For this review, take the finished solid that the model builds, in its own axes (mm). Round coordinates to 2 decimals unless told otherwise and drop trailing zeros. Order: outer loops, then holes, each group sorted by start corner. A loop starts at its lowest first (then second) coordinate and runs counter-clockwise, first axis right, second up. Notation, with made-up numbers: M 81.25,7.5 L 98.25,7.5 A14 cw 98.25,17.5 Z; hole C 70,87.5 d6. An arc over 180 degrees is marked long. Answer as a JSON object with one key per item and string values.
from build123d import *

# Parameters (mm, degrees)
BOSS_EXTRUDE1_DEPTH = 10
CUT_EXTRUDE1_REACH  = 96.868
SKETCH2_R           = 2.5


with BuildPart() as part:
    # Sketch1 → Boss-Extrude1 (new body)
    with BuildSketch(Plane.XY):
        Polygon((0, 0), (50, 0), (50, 80), (-40, 80), (-40, 40), align=None)
    extrude(amount=BOSS_EXTRUDE1_DEPTH)

    # Sketch2 → Cut-Extrude1 (cut, up to next)
    with BuildSketch(Plane.XY.offset(10), mode=Mode.PRIVATE) as cut_extrude1_sk1:
        with Locations((10, 10)):
            Circle(SKETCH2_R)
    cut_extrude1_tool1 = extrude(cut_extrude1_sk1.sketch, amount=-CUT_EXTRUDE1_REACH, mode=Mode.PRIVATE) & part.part
    # Sketch2 → Cut-Extrude1 (cut, up to next)
    with BuildSketch(Plane.XY.offset(10), mode=Mode.PRIVATE) as cut_extrude1_sk2:
        with Locations((30, 10)):
            Circle(SKETCH2_R)
    cut_extrude1_tool2 = extrude(cut_extrude1_sk2.sketch, amount=-CUT_EXTRUDE1_REACH, mode=Mode.PRIVATE) & part.part
    # Sketch2 → Cut-Extrude1 (cut, up to next)
    with BuildSketch(Plane.XY.offset(10), mode=Mode.PRIVATE) as cut_extrude1_sk3:
        with Locations((10, 30)):
            Circle(SKETCH2_R)
    cut_extrude1_tool3 = extrude(cut_extrude1_sk3.sketch, amount=-CUT_EXTRUDE1_REACH, mode=Mode.PRIVATE) & part.part
    # Sketch2 → Cut-Extrude1 (cut, up to next)
    with BuildSketch(Plane.XY.offset(10), mode=Mode.PRIVATE) as cut_extrude1_sk4:
        with Locations((30, 30)):
            Circle(SKETCH2_R)
    cut_extrude1_tool4 = extrude(cut_extrude1_sk4.sketch, amount=-CUT_EXTRUDE1_REACH, mode=Mode.PRIVATE) & part.part
    # Sketch2 → Cut-Extrude1 (cut, up to next)
    with BuildSketch(Plane.XY.offset(10), mode=Mode.PRIVATE) as cut_extrude1_sk5:
        with Locations((10, 50)):
            Circle(SKETCH2_R)
    cut_extrude1_tool5 = extrude(cut_extrude1_sk5.sketch, amount=-CUT_EXTRUDE1_REACH, mode=Mode.PRIVATE) & part.part
    # Sketch2 → Cut-Extrude1 (cut, up to next)
    with BuildSketch(Plane.XY.offset(10), mode=Mode.PRIVATE) as cut_extrude1_sk6:
        with Locations((30, 50)):
            Circle(SKETCH2_R)
    cut_extrude1_tool6 = extrude(cut_extrude1_sk6.sketch, amount=-CUT_EXTRUDE1_REACH, mode=Mode.PRIVATE) & part.part
    # Sketch2 → Cut-Extrude1 (cut, up to next)
    with BuildSketch(Plane.XY.offset(10), mode=Mode.PRIVATE) as cut_extrude1_sk7:
        with Locations((10, 70)):
            Circle(SKETCH2_R)
    cut_extrude1_tool7 = extrude(cut_extrude1_sk7.sketch, amount=-CUT_EXTRUDE1_REACH, mode=Mode.PRIVATE) & part.part
    # Sketch2 → Cut-Extrude1 (cut, up to next)
    with BuildSketch(Plane.XY.offset(10), mode=Mode.PRIVATE) as cut_extrude1_sk8:
        with Locations((30, 70)):
            Circle(SKETCH2_R)
    cut_extrude1_tool8 = extrude(cut_extrude1_sk8.sketch, amount=-CUT_EXTRUDE1_REACH, mode=Mode.PRIVATE) & part.part
    # Sketch2 → Cut-Extrude1 (cut, up to next)
    with BuildSketch(Plane.XY.offset(10), mode=Mode.PRIVATE) as cut_extrude1_sk9:
        with Locations((-30, 50)):
            Circle(SKETCH2_R)
    cut_extrude1_tool9 = extrude(cut_extrude1_sk9.sketch, amount=-CUT_EXTRUDE1_REACH, mode=Mode.PRIVATE) & part.part
    # Sketch2 → Cut-Extrude1 (cut, up to next)
    with BuildSketch(Plane.XY.offset(10), mode=Mode.PRIVATE) as cut_extrude1_sk10:
        with Locations((-10, 50)):
            Circle(SKETCH2_R)
    cut_extrude1_tool10 = extrude(cut_extrude1_sk10.sketch, amount=-CUT_EXTRUDE1_REACH, mode=Mode.PRIVATE) & part.part
    # Sketch2 → Cut-Extrude1 (cut, up to next)
    with BuildSketch(Plane.XY.offset(10), mode=Mode.PRIVATE) as cut_extrude1_sk11:
        with Locations((-30, 70)):
            Circle(SKETCH2_R)
    cut_extrude1_tool11 = extrude(cut_extrude1_sk11.sketch, amount=-CUT_EXTRUDE1_REACH, mode=Mode.PRIVATE) & part.part
    # Sketch2 → Cut-Extrude1 (cut, up to next)
    with BuildSketch(Plane.XY.offset(10), mode=Mode.PRIVATE) as cut_extrude1_sk12:
        with Locations((-10, 70)):
            Circle(SKETCH2_R)
    cut_extrude1_tool12 = extrude(cut_extrude1_sk12.sketch, amount=-CUT_EXTRUDE1_REACH, mode=Mode.PRIVATE) & part.part
    # Sketch2 → Cut-Extrude1 (cut, up to next)
    with BuildSketch(Plane.XY.offset(10), mode=Mode.PRIVATE) as cut_extrude1_sk13:
        with Locations((45, 10)):
            Circle(SKETCH2_R)
    cut_extrude1_tool13 = extrude(cut_extrude1_sk13.sketch, amount=-CUT_EXTRUDE1_REACH, mode=Mode.PRIVATE) & part.part
    # Sketch2 → Cut-Extrude1 (cut, up to next)
    with BuildSketch(Plane.XY.offset(10), mode=Mode.PRIVATE) as cut_extrude1_sk14:
        with Locations((45, 70)):
            Circle(SKETCH2_R)
    cut_extrude1_tool14 = extrude(cut_extrude1_sk14.sketch, amount=-CUT_EXTRUDE1_REACH, mode=Mode.PRIVATE) & part.part
    add(cut_extrude1_tool1.solids().sort_by_distance((10, 10, 10))[0], mode=Mode.SUBTRACT)
    add(cut_extrude1_tool2.solids().sort_by_distance((30, 10, 10))[0], mode=Mode.SUBTRACT)
    add(cut_extrude1_tool3.solids().sort_by_distance((10, 30, 10))[0], mode=Mode.SUBTRACT)
    add(cut_extrude1_tool4.solids().sort_by_distance((30, 30, 10))[0], mode=Mode.SUBTRACT)
    add(cut_extrude1_tool5.solids().sort_by_distance((10, 50, 10))[0], mode=Mode.SUBTRACT)
    add(cut_extrude1_tool6.solids().sort_by_distance((30, 50, 10))[0], mode=Mode.SUBTRACT)
    add(cut_extrude1_tool7.solids().sort_by_distance((10, 70, 10))[0], mode=Mode.SUBTRACT)
    add(cut_extrude1_tool8.solids().sort_by_distance((30, 70, 10))[0], mode=Mode.SUBTRACT)
    add(cut_extrude1_tool9.solids().sort_by_distance((-30, 50, 10))[0], mode=Mode.SUBTRACT)
    add(cut_extrude1_tool10.solids().sort_by_distance((-10, 50, 10))[0], mode=Mode.SUBTRACT)
    add(cut_extrude1_tool11.solids().sort_by_distance((-30, 70, 10))[0], mode=Mode.SUBTRACT)
    add(cut_extrude1_tool12.solids().sort_by_distance((-10, 70, 10))[0], mode=Mode.SUBTRACT)
    add(cut_extrude1_tool13.solids().sort_by_distance((45, 10, 10))[0], mode=Mode.SUBTRACT)
    add(cut_extrude1_tool14.solids().sort_by_distance((45, 70, 10))[0], mode=Mode.SUBTRACT)


solid = part.part
1) Add section A-A on x = 10. State the section outline as (y, z) points, and give its area (3 significant figures).
Geometry check:
{"outline": "M 0,0 L 7.5,0 L 7.5,10 L 0,10 Z; M 12.5,0 L 27.5,0 L 27.5,10 L 12.5,10 Z; M 32.5,0 L 47.5,0 L 47.5,10 L 32.5,10 Z; M 52.5,0 L 67.5,0 L 67.5,10 L 52.5,10 Z; M 72.5,0 L 80,0 L 80,10 L 72.5,10 Z", "area": "600 mm²"}
2) Add section B-B on y = 50. State the section outline as (x, z) points.
Geometry check:
{"outline": "M -40,0 L -32.5,0 L -32.5,10 L -40,10 Z; M -27.5,0 L -12.5,0 L -12.5,10 L -27.5,10 Z; M -7.5,0 L 7.5,0 L 7.5,10 L -7.5,10 Z; M 12.5,0 L 27.5,0 L 27.5,10 L 12.5,10 Z; M 32.5,0 L 50,0 L 50,10 L 32.5,10 Z"}
3) Insertion check: P1, Ø1.5, axis at x = -15.5, z = 7, coming from the -Y side; P2, Ø3, axis at x = -10, y = 50, coming from the -Z side. Each pin has a flat end and moves straight along its axis. Give the tip position at first contact, or say it passes through.
Geometry check:
{"P1": "stops at y = 14.75", "P2": "passes through"}
4) Add section C-C on y = 30. State the section outline as (x, z) points, and give its area (3 significant figures).
Geometry check:
{"outline": "M -30,0 L 7.5,0 L 7.5,10 L -30,10 Z; M 12.5,0 L 27.5,0 L 27.5,10 L 12.5,10 Z; M 32.5,0 L 50,0 L 50,10 L 32.5,10 Z", "area": "700 mm²"}
5) Add section D-D on x = 45. State the section outline as (y, z) points, and give its area (3 significant figures).
Geometry check:
{"outline": "M 0,0 L 7.5,0 L 7.5,10 L 0,10 Z; M 12.5,0 L 67.5,0 L 67.5,10 L 12.5,10 Z; M 72.5,0 L 80,0 L 80,10 L 72.5,10 Z", "area": "700 mm²"}
6) Mouldability with a two-part tool opening along Y and no side actions: class faces 1 (the flat face through (-20, 20, 5)), 2 (the flat face through (4, 41, 0)), 3 (the cylindrical face through (28.16, 51.69, 5.07)), 4 (the cylindrical face through (11.34, 32.11, 5.07)) as +Y half, -Y half, draft (parallel to the pull), parting line (faces both ways), or undercut.
Geometry check:
{"face 1": "-Y half", "face 2": "draft", "face 3": "undercut", "face 4": "undercut"}
7) For L1, parallel to Y at x = 10, z = 8; L2, parallel to Y at x = -10, z = 4.75; L3, parallel to Y at x = 8.5, z = 6.75, list the stretches that pass through material, from the lowest coordinate up.
Geometry check:
{"L1": "y = 0 to 7.5, 12.5 to 27.5, 32.5 to 47.5, 52.5 to 67.5, 72.5 to 80", "L2": "y = 10 to 47.5, 52.5 to 67.5, 72.5 to 80", "L3": "y = 0 to 8, 12 to 28, 32 to 48, 52 to 68, 72 to 80"}
